from build123d import *

# Parameters (mm, degrees)
F0_W     = 254
F0_H     = 254
F0_W_2   = 50.8
F0_H_2   = 50.8
F1_DEPTH = 76.2
F2_R     = 5.08


with BuildPart() as f1:
    # F0 (on Top) → F1 (new body)
    with BuildSketch(Plane.XY):
        with Locations((0.930347, 19.759098)):
            Rectangle(F0_W, F0_H)
        with Locations((-75.269653, -56.440902)):
            Rectangle(F0_W_2, F0_H_2, mode=Mode.SUBTRACT)
        with Locations((0.930347, -56.440902)):
            Rectangle(F0_W_2, F0_H_2, mode=Mode.SUBTRACT)
        with Locations((77.130347, -56.440902)):
            Rectangle(F0_W_2, F0_H_2, mode=Mode.SUBTRACT)
        with Locations((-75.269653, 19.759098)):
            Rectangle(F0_W_2, F0_H_2, mode=Mode.SUBTRACT)
        with Locations((-75.269653, 95.959098)):
            Rectangle(F0_W_2, F0_H_2, mode=Mode.SUBTRACT)
        with Locations((0.930347, 19.759098)):
            Rectangle(F0_W_2, F0_H_2, mode=Mode.SUBTRACT)
        with Locations((77.130347, 19.759098)):
            Rectangle(F0_W_2, F0_H_2, mode=Mode.SUBTRACT)
        with Locations((0.930347, 95.959098)):
            Rectangle(F0_W_2, F0_H_2, mode=Mode.SUBTRACT)
        with Locations((77.130347, 95.959098)):
            Rectangle(F0_W_2, F0_H_2, mode=Mode.SUBTRACT)
    extrude(amount=F1_DEPTH)

    # F2
    f2_edges = [f1.edges().sort_by_distance(p)[0] for p in [
        (-126.069653, 19.759098, 76.2),
        (0.930347, -107.240902, 76.2),
        (-126.069653, -107.240902, 38.1),
        (0.930347, -107.240902, 0),
        (-126.069653, 19.759098, 0),
        (-126.069653, 146.759098, 38.1),
        (0.930347, 146.759098, 76.2),
        (127.930347, 19.759098, 76.2),
        (-75.269653, -31.040902, 76.2),
        (-49.869653, -56.440902, 76.2),
        (-75.269653, -81.840902, 76.2),
        (-100.669653, -56.440902, 76.2),
        (-24.469653, -56.440902, 76.2),
        (0.930347, -31.040902, 76.2),
        (26.330347, -56.440902, 76.2),
        (0.930347, -81.840902, 76.2),
        (77.130347, -31.040902, 76.2),
        (102.530347, -56.440902, 76.2),
        (77.130347, -81.840902, 76.2),
        (51.730347, -56.440902, 76.2),
        (-75.269653, 45.159098, 76.2),
        (-49.869653, 19.759098, 76.2),
        (-75.269653, -5.640902, 76.2),
        (-100.669653, 19.759098, 76.2),
        (-100.669653, 95.959098, 76.2),
        (-75.269653, 121.359098, 76.2),
        (-49.869653, 95.959098, 76.2),
        (-75.269653, 70.559098, 76.2),
        (-24.469653, 19.759098, 76.2),
        (0.930347, 45.159098, 76.2),
        (26.330347, 19.759098, 76.2),
        (0.930347, -5.640902, 76.2),
        (77.130347, 45.159098, 76.2),
        (102.530347, 19.759098, 76.2),
        (77.130347, -5.640902, 76.2),
        (51.730347, 19.759098, 76.2),
        (-24.469653, 95.959098, 76.2),
        (0.930347, 121.359098, 76.2),
        (26.330347, 95.959098, 76.2),
        (0.930347, 70.559098, 76.2),
        (77.130347, 121.359098, 76.2),
        (102.530347, 95.959098, 76.2),
        (77.130347, 70.559098, 76.2),
        (51.730347, 95.959098, 76.2),
        (127.930347, -107.240902, 38.1),
        (127.930347, 146.759098, 38.1),
        (127.930347, 19.759098, 0),
        (0.930347, 146.759098, 0),
    ]]
    fillet(f2_edges, radius=F2_R)


solid = f1.part
Build history of the part. All positions in model axes, mm. Give positions to 0.01 mm unless a question says otherwise; leave off trailing zeros. Order: outer loops, then holes, each group sorted by start corner. A loop starts at its lowest first (then second) coordinate and runs counter-clockwise, first axis right, second up. Notation, with made-up numbers: M 78.5,48 L 108.5,48 A11 cw 108.5,58 Z; hole C 66.5,55 d11. An arc over 180 degrees is marked long. Put each result on its own line as item: value.
Item 1: Probe line 1 (Y direction, x = 75.5, z = 54.5); line 2 (X direction, y = -57, z = 70); line 3 (Y direction, x = 18, z = 4). List the from-to ranges inside material, lowest first. Write a range as [from, to].
From the geometry:
line 1: y = [-107.24, -81.84], [-31.04, -5.64], [45.16, 70.56], [121.36, 146.76]
line 2: x = [-126.07, -100.67], [-49.87, -24.47], [26.33, 51.73], [102.53, 127.93]
line 3: y = [-107.12, -81.84], [-31.04, -5.64], [45.16, 70.56], [121.36, 146.64]
Item 2: Two-plate mould, pull along X, no slides. Class faces 1 (the flat face through (0, -16, 76.2)), 2 (the flat face through (-126.07, 18, 38)), 3 (the flat face through (-24.47, 96, 35)): +X half, -X half, draft (parallel to the pull), parting line (faces both ways), or undercut.
From the geometry:
face 1: draft
face 2: -X half
face 3: undercut
Item 3: Slice it at C-C, the plane z = 41. Give the number of separate pieces and of enclosed holes in the cut face, plus the area to 3 significant figures.
From the geometry:
separate pieces: 1
enclosed holes: 9
area: 41,300 mm2
Item 4: Flat gauge pin, fed straight in: pin 1 Ø1.5 at (x, y) = (49, 114) entering from +Z. Where does the tip first touch, or does it go through?
From the geometry:
pin 1: stops at z = 75.94
Item 5: Slice it at A-A, the plane x = -79. Write the cut outline in (y, z), plus the area to 3 significant figures.
From the geometry:
outline: M -107.24,5.08 A5.08 ccw -102.16,0 L -81.84,0 L -81.84,71.12 A5.08 ccw -86.92,76.2 L -102.16,76.2 A5.08 ccw -107.24,71.12 Z; M -31.04,0 L -5.64,0 L -5.64,71.12 A5.08 ccw -10.72,76.2 L -25.96,76.2 A5.08 ccw -31.04,71.12 Z; M 45.16,0 L 70.56,0 L 70.56,71.12 A5.08 ccw 65.48,76.2 L 50.24,76.2 A5.08 ccw 45.16,71.12 Z; M 121.36,0 L 141.68,0 A5.08 ccw 146.76,5.08 L 146.76,71.12 A5.08 ccw 141.68,76.2 L 126.44,76.2 A5.08 ccw 121.36,71.12 Z
area: 7,690 mm2
Item 6: Slice it at B-B, the plane y = -72.5. Write the cut outline in (x, z).
From the geometry:
outline: M -126.07,5.08 A5.08 ccw -120.99,0 L -100.67,0 L -100.67,71.12 A5.08 ccw -105.75,76.2 L -120.99,76.2 A5.08 ccw -126.07,71.12 Z; M -49.87,0 L -24.47,0 L -24.47,71.12 A5.08 ccw -29.55,76.2 L -44.79,76.2 A5.08 ccw -49.87,71.12 Z; M 26.33,0 L 51.73,0 L 51.73,71.12 A5.08 ccw 46.65,76.2 L 31.41,76.2 A5.08 ccw 26.33,71.12 Z; M 102.53,0 L 122.85,0 A5.08 ccw 127.93,5.08 L 127.93,71.12 A5.08 ccw 122.85,76.2 L 107.61,76.2 A5.08 ccw 102.53,71.12 Z
